Job drawing, mm, ordinate dimensions from the low corner. One solid piece. A direction names the side the tool comes from. Round coordinates to 2 decimals unless told otherwise and drop trailing zeros. Order: outer loops, then holes, each group sorted by start corner. A loop starts at its lowest first (then second) coordinate and runs counter-clockwise, first axis right, second up. Notation, with made-up numbers: (10.5, 10) -> (26.5, 10) arc R20 cw to (26.5, 33) -> close; hole circle Ø9 at (77, 35.5). An arc over 180 degrees is marked (long way). Use CSV: the item, a comma, the result in double quotes.
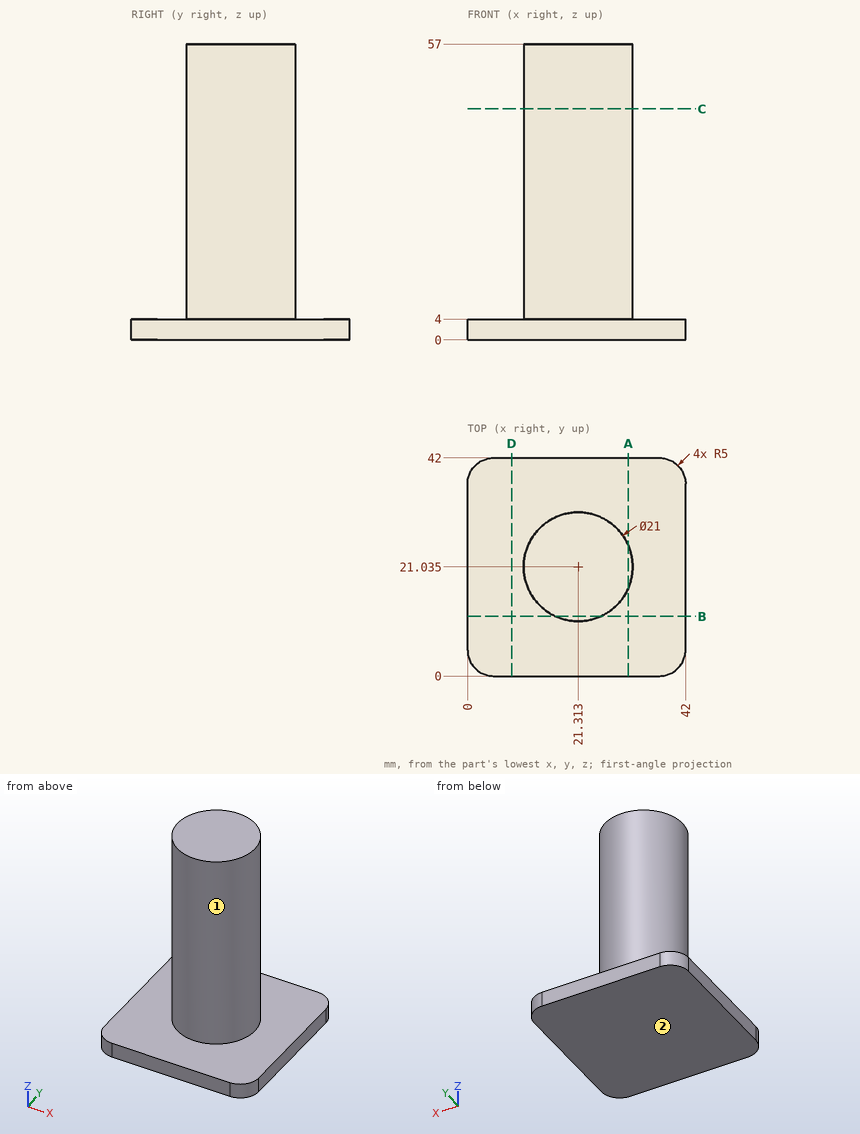
(1) Cut at B-B, the plane y = 11.5. Give the cut face in (x, z).
Reply:
outline,"(0, 0) -> (42, 0) -> (42, 4) -> (25.71, 4) -> (25.71, 57) -> (16.92, 57) -> (16.92, 4) -> (0, 4) -> close"
(2) Which spindle directions (+Z, -Z, +X, -X, +Y, -Y) get a long thin tool onto all of the face, cutting with end or side? Do the marked faces 1 and 2. Say none if no direction does.
Reply:
face 1,"+Z"
face 2,"-Z, +X, -X, +Y, -Y"
(3) Cut at D-D, the plane x = 8.5. Give the cut face in (y, z).
Reply:
outline,"(0, 0) -> (42, 0) -> (42, 4) -> (0, 4) -> close"
(4) Cut at A-A, the plane x = 31. Give the cut face in (y, z), then the cut area to 3 significant figures.
Reply:
outline,"(0, 0) -> (42, 0) -> (42, 4) -> (25.09, 4) -> (25.09, 57) -> (16.98, 57) -> (16.98, 4) -> (0, 4) -> close"
area,"597 mm2"
(5) Drop flat-ended pins along their axis: P1, Ø6, axis at y = 22.5, z = 13, coming from the +X side; P2, Ø3, axis at x = 17.5, z = 43, coming from the +Y side; P3, Ø12, axis at x = 25, z = 19.5, coming from the -Y side (3 decimals). Give the stop position or say it passes through.
Reply:
P1,"x = 31.81"
P2,"y = 31.28"
P3,"y = 10.535"
(6) Probe probe 1 along Z at (x, y) = (21, 3); probe 2 along X at (y, z) = (16, 44); probe 3 along X at (y, z) = (16.5, 17). List the from-to ranges inside material, lowest first. Write a range as [from, to].
Reply:
probe 1,"[0, 4]"
probe 2,"[12.1, 30.53]"
probe 3,"[11.84, 30.78]"
(7) Cut at C-C, the plane z = 44.5. Give the cut face in (x, y) (1 decimal).
Reply:
outline,"circle Ø21 at (21.3, 21)"
